Source: CAD feature listing. Evaluate the final solid. Frame: model axes, mm. Face numbers are marked on the shaded views. A direction names the side the tool comes from. Give positions to 0.01 mm unless a question says otherwise; leave off trailing zeros. Loops run counter-clockwise (first coordinate to the right, second up) from the corner with the lowest first, then second, coordinate; pieces in that order, holes last. Notation, with made-up numbers: (48, 74) -> (59, 74) arc R19 cw to (59, 80) -> close; hole circle Ø9 at (-4.5, 6.5). An arc over 180 degrees is marked (long way). Answer as a JSON object with one key per item and string values. Group by question number.
Autodesk Inventor part; units mm, degrees
ref_plane "YZ Plane" through (0, 0, 0) normal (1, 0, 0) x (0, 1, 0)
ref_plane "XZ Plane" through (0, 0, 0) normal (0, 1, 0) x (-1, 0, 0)
ref_plane "XY Plane" through (0, 0, 0) normal (0, 0, 1) x (1, 0, 0)
sketch "Boceto1" plane through (0, 0, 0) normal (0, 1, 0) x (-1, 0, 0)
  line L0 (0, 0) -> (100, 0)
  line L1 (100, 0) -> (100, -31.85)
  line L2 (100, -31.85) -> (-100, -31.85)
  line L3 (-100, -31.85) -> (-100, 31.85)
  line L4 (-100, 31.85) -> (100, 31.85)
  line L5 (100, 31.85) -> (100, -31.85)
  dimension "d0" = 100
  dimension "d1" = 31.85
  dimension "d2" = 200
  dimension "d3" = 63.7
extrude "Extrusión1" add sketch "Boceto1" along normal blind 76.62
sketch "Boceto2" plane through (0, 76.62, 0) normal (0, 1, 0) x (1, 0, 0)
  line L0 (-100, 31.85) -> (-100, -31.85)
  line L1 (-100, 0) -> (-97, 0)
  line L2 (-97, 0) -> (-97, 29.85)
  line L3 (-97, 29.85) -> (-79.76, 29.85)
  line L4 (-97, 29.85) -> (-79.76, 29.85)
  line L5 (-79.76, 29.85) -> (-79.76, -29.85)
  line L6 (-79.76, -29.85) -> (-97, -29.85)
  line L7 (-97, -29.85) -> (-97, 29.85)
  line L8 (-79.76, 0) -> (-76.76, 0)
  line L9 (-76.76, 0) -> (-76.76, 29.85)
  line L10 (-76.76, 29.85) -> (-59.52, 29.85)
  line L11 (-59.52, 29.85) -> (-59.52, -29.85)
  line L12 (-59.52, -29.85) -> (-76.76, -29.85)
  line L13 (-76.76, -29.85) -> (-76.76, 29.85)
  line L14 (-59.52, 0) -> (-56.52, 0)
  line L15 (-56.52, 0) -> (-56.52, 29.85)
  line L16 (-56.52, 29.85) -> (-39.28, 29.85)
  line L17 (-39.28, 29.85) -> (-39.28, -29.85)
  line L18 (-39.28, -29.85) -> (-56.52, -29.85)
  line L19 (-56.52, -29.85) -> (-56.52, 29.85)
  line L20 (-39.28, 0) -> (-36.28, 0)
  line L21 (-36.28, 0) -> (-36.28, 29.85)
  line L22 (-36.28, 29.85) -> (-19.04, 29.85)
  line L23 (-19.04, 29.85) -> (-19.04, -29.85)
  line L24 (-19.04, -29.85) -> (-36.28, -29.85)
  line L25 (-36.28, -29.85) -> (-36.28, 29.85)
  line L26 (-19.04, 0) -> (-16.04, 0)
  line L27 (-16.04, 0) -> (-16.04, 29.85)
  line L28 (-16.04, 29.85) -> (1.2, 29.85)
  line L29 (1.2, 29.85) -> (1.2, -29.85)
  line L30 (1.2, -29.85) -> (-16.04, -29.85)
  line L31 (-16.04, -29.85) -> (-16.04, 29.85)
  line L32 (1.2, 0) -> (2.7, 0)
  line L33 (2.7, 0) -> (2.7, 9.0784)
  line L34 (82.16, 0) -> (82.16, 29.85)
  line L35 (82.16, 29.85) -> (64.92, 29.85)
  line L36 (64.92, 29.85) -> (64.92, -29.85)
  line L37 (64.92, -29.85) -> (82.16, -29.85)
  line L38 (82.16, -29.85) -> (82.16, 29.85)
  line L39 (64.92, 0) -> (61.92, 0)
  line L40 (61.92, 0) -> (61.92, 29.85)
  line L41 (61.92, 29.85) -> (44.68, 29.85)
  line L42 (44.68, 29.85) -> (44.68, -29.85)
  line L43 (44.68, -29.85) -> (61.92, -29.85)
  line L44 (61.92, -29.85) -> (61.92, 29.85)
  line L45 (44.68, 0) -> (41.68, 0)
  line L46 (41.68, 0) -> (41.68, 29.85)
  line L47 (41.68, 29.85) -> (24.44, 29.85)
  line L48 (24.44, 29.85) -> (24.44, -29.85)
  line L49 (24.44, -29.85) -> (41.68, -29.85)
  line L50 (41.68, -29.85) -> (41.68, 29.85)
  line L51 (24.44, 0) -> (21.44, 0)
  line L52 (21.44, 0) -> (21.44, 29.85)
  line L53 (21.44, 29.85) -> (4.2, 29.85)
  line L54 (4.2, 29.85) -> (4.2, -29.85)
  line L55 (4.2, -29.85) -> (21.44, -29.85)
  line L56 (21.44, -29.85) -> (21.44, 29.85)
  line L57 (82.16, 0) -> (85.16, 0)
  line L58 (85.16, 0) -> (85.16, 31.85)
  line L59 (100, -31.85) -> (100, 31.85)
  line L60 (85.16, 31.85) -> (100, 31.85)
  line L61 (100, 31.85) -> (100, -31.85)
  line L62 (100, -31.85) -> (85.16, -31.85)
  line L63 (85.16, -31.85) -> (85.16, 31.85)
  point P0 (0, 0)
  point P1 (5.4, 0)
  point P2 (4.2, 0)
  dimension "d6" = 3
  dimension "d7" = 29.85
  dimension "d8" = 17.24
  dimension "d9" = 17.24
  dimension "d10" = 59.7
  dimension "d11" = 3
  dimension "d12" = 17.24
  dimension "d13" = 59.7
  dimension "d14" = 3
  dimension "d15" = 17.24
  dimension "d16" = 59.7
  dimension "d17" = 3
  dimension "d18" = 17.24
  dimension "d19" = 59.7
  dimension "d20" = 3
  dimension "d21" = 17.24
  dimension "d22" = 59.7
  dimension "d23" = 1.5
  dimension "d24" = 3
extrude "Extrusión2" cut sketch "Boceto2" against normal blind 76.62
sketch "Boceto3" plane through (64.92, 76.62, 29.85) normal (1, 0, 0) x (0, 0, -1)
  line L0 (-2, 0) -> (61.7, 0)
  line L1 (-2, 0) -> (29.85, 0)
  line L2 (29.85, 0) -> (19.85, 0)
  point P0 (29.85, -76.62)
  dimension "d27" = 31.85
  dimension "d28" = 10
sketch "Boceto4" plane through (0, 0, 0) normal (0, -1, 0) x (1, 0, 0)
  line L0 (-100, -31.85) -> (-100, 31.85)
  line L1 (-100, 31.85) -> (85.16, 31.85)
  line L2 (85.16, 31.85) -> (85.16, -31.85)
  line L3 (85.16, -31.85) -> (-100, -31.85)
  line L4 (-100, -31.85) -> (-100, 31.85)
  point P0 (0, 0)
extrude "Extrusión3" add sketch "Boceto4" along normal blind 3
sketch "Boceto5" plane through (0, 76.62, 0) normal (0, 1, 0) x (1, 0, 0)
  line L0 (85.16, -31.85) -> (85.16, 31.85)
  line L1 (-100, -31.85) -> (85.16, -31.85)
  line L2 (85.16, -31.85) -> (85.16, 31.85)
  line L3 (85.16, 31.85) -> (-100, 31.85)
  line L4 (-100, 31.85) -> (-100, -31.85)
  point P0 (0, 0)
extrude "Extrusión4" cut sketch "Boceto5" against normal blind 20
sketch "Boceto6" plane through (85.16, -3, -31.85) normal (0, 0, -1) x (-1, 0, 0)
  point P0 (85.16, 3)
equation "\"d3\" = 2 * d1"
equation "\"d9\" = d8"
equation "\"d10\" = 2 * d7"
equation "\"d12\" = d8"
equation "\"d13\" = 2 * d7"
equation "\"d15\" = d8"
equation "\"d16\" = 2 * d7"
equation "\"d18\" = d8"
equation "\"d19\" = 2 * d7"
equation "\"d21\" = d8"
equation "\"d22\" = 2 * d7"
properties part number "Base_Principal"
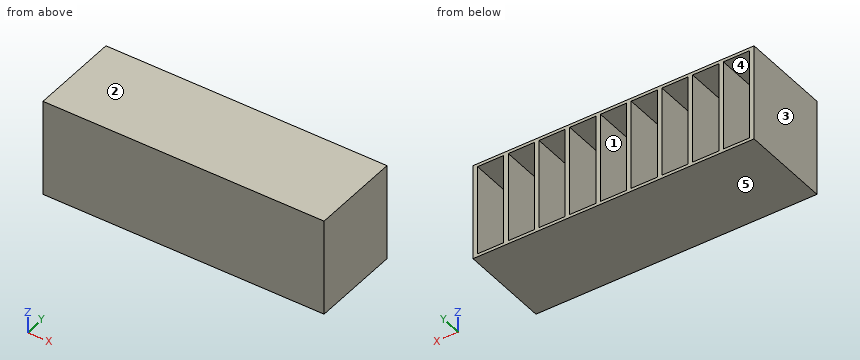
(1) Section query A-A on x = 52. Return the cut outline in (y, z), plus the area to 3 significant figures.
(2) First-contact query: pin 1 (8.5 mm diameter, centred on x = 12, z = 10, fed in from +Y). Flat tip, straight axial feed; report the tip coordinate or a pass-through.
(3) Access query for the marked faces 4 and 5. Directions: +Z, -Z, +X, -X, +Y, -Y. A direction counts if a zero-diameter tool reaches every point of the face in a straight line with its end or side. Return the directions, or none.
(4) Mould query, pull axis X, two halves, no side actions, for the marked faces 1, 2 and 3. Classes: pulls with the +X half, pulls with the -X half, needs draft (parallel to the pull), parting line crosses it, or undercut.
(5) Section query B-B on y = 48.5. State how many separate pieces and enclosed holes the cut face has, plus the area to 3 significant figures.
(6) Material intervals for line 1 (Z direction, x = -64.5, y = 2); line 2 (Y direction, x = -40, z = -27), sorted ascending. Write a range as from..to.
Result:
{
 "1": {"outline": "(-3, -31.85) -> (56.62, -31.85) -> (56.62, -29.85) -> (0, -29.85) -> (0, 29.85) -> (56.62, 29.85) -> (56.62, 31.85) -> (-3, 31.85) -> close", "area": "418 mm²"},
 "2": {"pin 1": "y = 0"},
 "3": {"face 4": "+Y", "face 5": "-Z, +X, -X, +Y, -Y"},
 "4": {"face 1": "undercut", "face 2": "needs draft", "face 3": "pulls with the -X half"},
 "5": {"separate pieces": "1", "enclosed holes": "9", "area": "2,530 mm²"},
 "6": {"line 1": "-31.85..-29.85, 29.85..31.85", "line 2": "-3..0"}
}
